Design review of the part built by this model. Coordinates are the model's own, in mm. Give positions to 0.01 mm unless a question says otherwise; leave off trailing zeros. Loops run counter-clockwise (first coordinate to the right, second up) from the corner with the lowest first, then second, coordinate; pieces in that order, holes last.
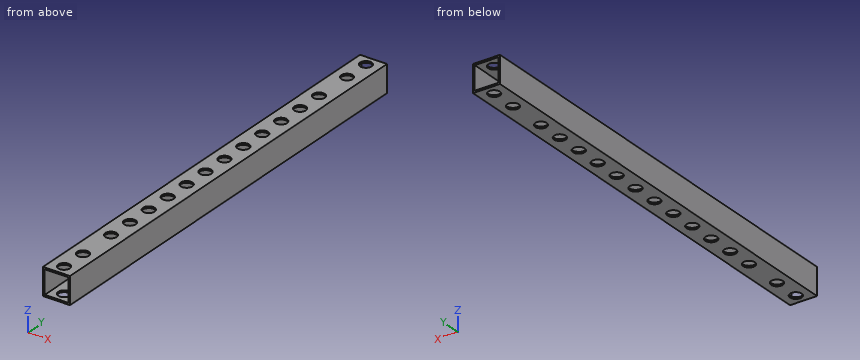
from build123d import *

# Parameters (mm, degrees)
SKETCH1_W                       = 25.4
SKETCH1_H                       = 25.4
SKETCH1_W_2                     = 22.225
SKETCH1_H_2                     = 22.225
EXTRUDE_THIN1_DEPTH             = 419.1
M10_CLEARANCE_HOLE1_D           = 11
M10_CLEARANCE_HOLE1_CSINK_D     = 11.05
M10_CLEARANCE_HOLE1_CSINK_ANGLE = 90
M10_CLEARANCE_HOLE2_D           = 11
M10_CLEARANCE_HOLE2_CSINK_D     = 11.05
M10_CLEARANCE_HOLE2_CSINK_ANGLE = 90
LPATTERN2_COUNT                 = 6
LPATTERN2_PITCH                 = 25
LPATTERN2_COL_COUNT             = 6
LPATTERN2_COL_PITCH             = 25


with BuildPart() as part:
    # Sketch1 → Extrude-Thin1 (new body)
    with BuildSketch(Plane(origin=(0, 0, 0), x_dir=(1, 0, 0), z_dir=(0, 1, 0))):
        Rectangle(SKETCH1_W, SKETCH1_H)
        Rectangle(SKETCH1_W_2, SKETCH1_H_2, mode=Mode.SUBTRACT)
    extrude(amount=EXTRUDE_THIN1_DEPTH)

    # M10 Clearance Hole1 (through all)
    with Locations(Plane(origin=(0, 0, -12.7), x_dir=(-1, 0, 0), z_dir=(0, 0, -1))):
        with Locations((0, 409.1), (0, 384.1), (0, 35), (0, 10)):
            CounterSinkHole(M10_CLEARANCE_HOLE1_D / 2, M10_CLEARANCE_HOLE1_CSINK_D / 2, counter_sink_angle=M10_CLEARANCE_HOLE1_CSINK_ANGLE)

    # M10 Clearance Hole2 (through all)
    with Locations(Plane(origin=(0, 0, -12.7), x_dir=(-1, 0, 0), z_dir=(0, 0, -1))):
        with Locations((0, 197.05), (0, 222.05)):
            m10_clearance_hole2 = CounterSinkHole(M10_CLEARANCE_HOLE2_D / 2, M10_CLEARANCE_HOLE2_CSINK_D / 2, counter_sink_angle=M10_CLEARANCE_HOLE2_CSINK_ANGLE)

    # LPattern2: M10 Clearance Hole2 ×6
    with Locations(*[(0, i * LPATTERN2_PITCH, 0) for i in range(1, LPATTERN2_COUNT)]):
        add(m10_clearance_hole2, mode=Mode.SUBTRACT)

    # LPattern2 col: M10 Clearance Hole2 ×6
    with Locations(*[(0, -i * LPATTERN2_COL_PITCH, 0) for i in range(1, LPATTERN2_COL_COUNT)]):
        add(m10_clearance_hole2, mode=Mode.SUBTRACT)


solid = part.part
Q1. Take a section at D-D (x = -0.75). Give the number of separate pieces and of enclosed holes in the cut face, plus the area to 3 significant figures.
Results:
separate pieces: 34
enclosed holes: 0
area: 777 mm2
Q2. Take a section at A-A (z = 2.75). Give the boundary of the cut face in (x, y).
Results:
outline: (-12.7, 0) - (-11.11, 0) - (-11.11, 419.1) - (-12.7, 419.1) - close; (11.11, 0) - (12.7, 0) - (12.7, 419.1) - (11.11, 419.1) - close
Q3. Wall thickness on line 1 (Z direction, x = -6.75, y = 113.5); line 2 (X direction, y = 272.05, z = 11.85): over which ranges is each line inside the solid? List them lowest first.
Results:
line 1: z = -12.7 to -11.11, 11.11 to 12.7
line 2: x = -12.7 to -5.5, 5.5 to 12.7
Q4. Take a section at C-C (y = 87). Give the boundary of the cut face in (x, z), plus the area to 3 significant figures.
Results:
outline: (-12.7, -12.7) - (12.7, -12.7) - (12.7, 12.7) - (-12.7, 12.7) - close; hole (-11.11, -11.11) - (11.11, -11.11) - (11.11, 11.11) - (-11.11, 11.11) - close
area: 151 mm2
